from build123d import *

# Parameters (mm, degrees)
F1_DEPTH = 500


with BuildPart() as f1:
    # F0 (on Front) → F1 (new body)
    with BuildSketch(Plane.XZ):
        Polygon((-252.215505, 381), (-284.065813, 381), (-278.574283, 363), (-273.035955, 344.846608), (-167.828424, 0), (-240.610838, -381), (240.610838, -381), (167.828424, 0), (284.065813, 381), align=None)
        Polygon((-149.312886, 0.994866), (-259.755226, 363), (259.755226, 363), (149.312886, 0.994866), (218.84681, -363), (-218.84681, -363), align=None, mode=Mode.SUBTRACT)
        with BuildLine():
            Line((-287.202322, 381), (-284.065813, 381))
            Line((-284.065813, 381), (-252.215505, 381))
            Line((-252.215505, 381), (-252.215505, 382))
            ThreePointArc((-252.215505, 382), (-252.801291, 383.414214), (-254.215505, 384))
            Line((-254.215505, 384), (-285.416401, 384))
            ThreePointArc((-285.416401, 384), (-287.023763, 383.19012), (-287.329356, 381.416386))
            Line((-287.329356, 381.416386), (-287.202322, 381))
        make_face()
        with BuildLine():
            Line((-278.574283, 363), (-284.065813, 381))
            Line((-284.065813, 381), (-287.202322, 381))
            Line((-287.202322, 381), (-276.489001, 345.884142))
            ThreePointArc((-276.489001, 345.884142), (-275.516032, 344.702416), (-273.992432, 344.554801))
            Line((-273.992432, 344.554801), (-273.035955, 344.846608))
            Line((-273.035955, 344.846608), (-278.574283, 363))
        make_face()
    extrude(amount=F1_DEPTH)


solid = f1.part
Can you work these out from the model? Positions are in its coordinate system, mm. A direction names the side the tool comes from. Give positions to 0.01 mm unless a question says otherwise; leave off trailing zeros. Order: outer loops, then holes, each group sorted by start corner. A loop starts at its lowest first (then second) coordinate and runs counter-clockwise, first axis right, second up. Notation, with made-up numbers: M 19,74 L 41,74 A27 cw 41,102 Z; hole C 72,74 d8. An arc over 180 degrees is marked long. One line per question, with ' | ' between items.
Item 1: Suppose I cut it at B-B, the plane y = -157.5. Write out the boundary of the cut face in (x, z).
Answer block:
outline: M -287.33,381.42 L -287.2,381 L -276.49,345.88 A2 ccw -273.99,344.55 L -273.04,344.85 L -167.83,0 L -240.61,-381 L 240.61,-381 L 167.83,0 L 284.07,381 L -252.22,381 L -252.22,382 A2 ccw -254.22,384 L -285.42,384 A2 ccw Z; hole M -259.76,363 L -149.31,0.99 L -218.85,-363 L 218.85,-363 L 149.31,0.99 L 259.76,363 Z
Item 2: Suppose I cut it at D-D, the plane x = -231. Write out the boundary of the cut face in (y, z), then the cut area to 3 significant figures.
Answer block:
outline: M -500,-381 L 0,-381 L 0,-330.69 L -500,-330.69 Z; M -500,207.06 L 0,207.06 L 0,268.75 L -500,268.75 Z; M -500,363 L 0,363 L 0,381 L -500,381 Z | area: 65,000 mm2
Item 3: Suppose I cut it at A-A, the plane x = 21. Write out the boundary of the cut face in (y, z).
Answer block:
outline: M -500,-381 L 0,-381 L 0,-363 L -500,-363 Z; M -500,363 L 0,363 L 0,381 L -500,381 Z
Item 4: For faces 4 (the face through (-203.71, -246.5, -187.83)), 5 (the face through (20, -246, 381)), 6 (the face through (3, -246, -363)), 7 (the face through (204.73, -246.5, -193.17)), which set-ups out of +Z, -Z, +X, -X, +Y, -Y let a thin tool reach every point of the face, with its end or its side?
Answer block:
face 4: -X, +Y, -Y | face 5: +Z, +X, +Y, -Y | face 6: +Y, -Y | face 7: +X, +Y, -Y
Item 5: I'm going to push flat-ended pins straight in: pin 1 Ø4 at (y, z) = (-319.5, 247.5) entering from -X; pin 2 Ø12 at (y, z) = (-312.5, 197.5) entering from +X; pin 3 Ø12 at (y, z) = (-286.5, -205) entering from -X. Where does each tip first touch, or does it pass through?
Answer block:
pin 1: stops at x = -243.95 | pin 2: stops at x = 229.91 | pin 3: stops at x = -208.14
Item 6: Please list where these lines run through material, in increasing order: L1, parallel to Z at x = 102, y = -27.5; L2, parallel to X at y = -428.5, z = -225; L3, parallel to X at y = -257, z = 139.
Answer block:
L1: z = -381 to -363, 363 to 381 | L2: x = -210.81 to -192.48, 192.48 to 210.81 | L3: x = -210.24 to -191.42, 191.42 to 210.24
Item 7: We'd pull the mould along Z, two halves only. Please class faces 1 (the face through (-3, -246, -381)), 2 (the face through (-221.17, -246.5, 174.84)), 3 (the face through (-151, -500, 3)): released by +Z, released by -Z, zero draft, split by the parting line, or undercut.
Answer block:
face 1: released by -Z | face 2: undercut | face 3: zero draft
Item 8: Suppose I cut it at C-C, the plane z = 232. Write out the boundary of the cut face in (x, y), then the cut area to 3 significant figures.
Answer block:
outline: M -238.61,-500 L -219.79,-500 L -219.79,0 L -238.61,0 Z; M 219.79,-500 L 238.61,-500 L 238.61,0 L 219.79,0 Z | area: 18,800 mm2
